Can you work these out from the drawing? Everything is in mm from the part's minimum corner. A direction names the side the tool comes from. Give positions to 0.01 mm unless a question says otherwise; leave off trailing zeros. Loops run counter-clockwise (first coordinate to the right, second up) from the corner with the lowest first, then second, coordinate; pieces in that order, holes last. Notation, with made-up numbers: (85.5, 47.5) - (133.5, 47.5) arc R32 cw to (133.5, 75.5) - close; hole circle Ø2 at (29.5, -39.5). An arc over 180 degrees is marked (long way). Write each question's results on one line, items separated by ' | '. Start each with the question number.
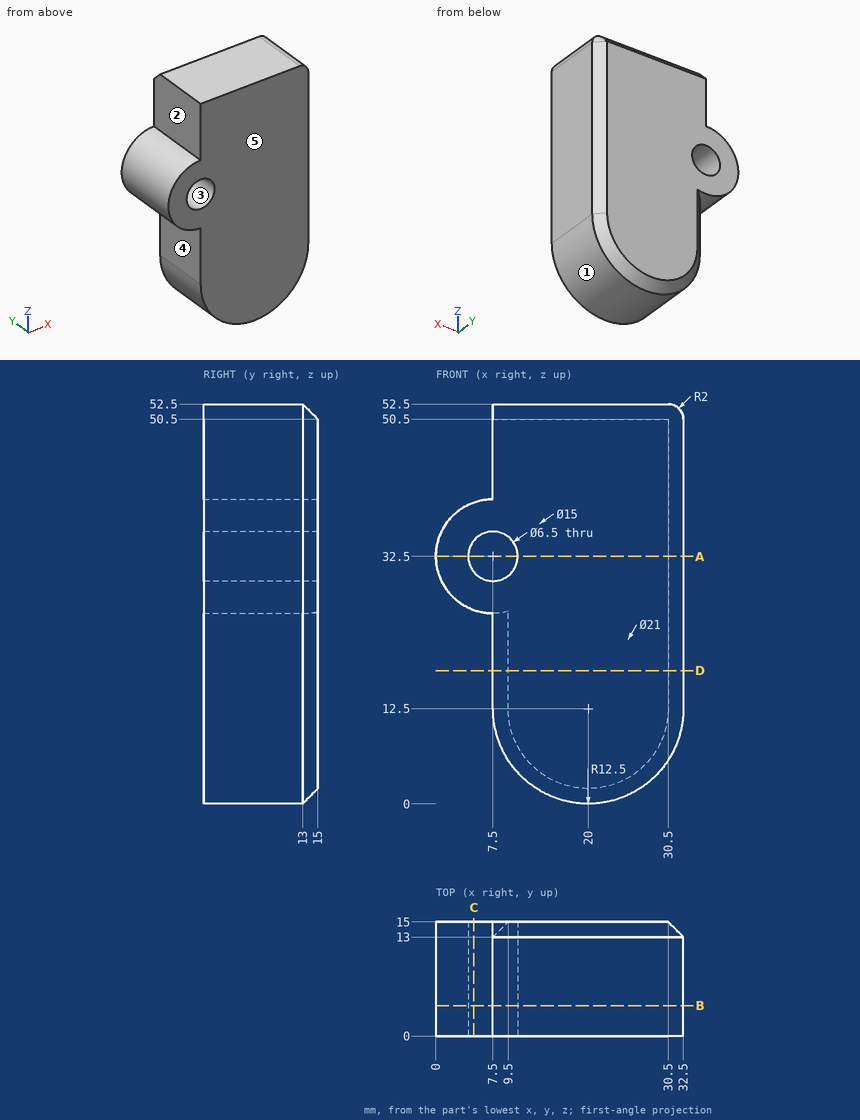
Q1. I want a section at B-B, the plane y = 4. List the corners of the cut face in (x, z) for me, then the cut area to 3 significant figures.
Q2. I want a section at C-C, the plane x = 5. List the corners of the cut face in (y, z) for me.
Q3. If we mould it in two halves opening along Z, with no side actions, what happens to the marked faces 1, 2 and 3? For each: +Z half, -Z half, draft (parallel to the pull), parting line (faces both ways), or undercut.
Q4. I need wall thicknesses on L1, parallel to X at y = 11.75, z = 32.5; L2, parallel to Z at x = 6, y = 3.25; L3, parallel to X at y = 8.75, z = 12. Which ranges of each line are inside material? Lowest first, please. Write a range as from..to.
Q5. I want a section at D-D, the plane z = 17.5. List the corners of the cut face in (x, y) for me, then the cut area to 3 significant figures.
Q6. I want a section at A-A, the plane z = 32.5. List the corners of the cut face in (x, y) for me, then the cut area to 3 significant figures.
Q7. Which directions (+Z, -Z, +X, -X, +Y, -Y) give clear straight access to the entire face, cutting with the end or side of a thin tool? Please do the marked faces 4 and 5.
Q8. I'm going to push flat-ended pins straight in: pin 1 Ø5 at (y, z) = (3, 9.5) entering from +X; pin 2 Ø4 at (y, z) = (7.5, 47) entering from -X. Where does each tip first touch, or does it pass through?
Conclusion:
1) outline: (7.5, 12.5) arc R12.5 ccw to (32.5, 12.5) - (32.5, 50.5) arc R2 ccw to (30.5, 52.5) - (7.5, 52.5) - (7.5, 40) arc R7.5 ccw to (7.5, 25) - close; hole circle Ø6.5 at (7.5, 32.5) | area: 1,300 mm^2
2) outline: (0, 25.43) - (15, 25.43) - (15, 30.42) - (0, 30.42) - close; (0, 34.58) - (15, 34.58) - (15, 39.57) - (0, 39.57) - close
3) face 1: -Z half | face 2: draft | face 3: undercut
4) L1: 0..4.25, 10.75..32.5 | L2: 25.15..29.62, 35.38..39.85 | L3: 7.51..32.49
5) outline: (7.5, 0) - (32.5, 0) - (32.5, 13) - (30.5, 15) - (9.5, 15) - (7.5, 13) - close | area: 371 mm^2
6) outline: (0, 0) - (4.25, 0) - (4.25, 15) - (0, 15) - close; (10.75, 0) - (32.5, 0) - (32.5, 13) - (30.5, 15) - (10.75, 15) - close | area: 388 mm^2
7) face 4: -Z, -X, +Y, -Y | face 5: +Z, -Z, +X, -X, -Y
8) pin 1: x = 32.49 | pin 2: x = 7.5
